Read the model definition and answer for the solid it produces. Units are mm, in the model's axes. Give positions to 0.01 mm unless a question says otherwise; leave off trailing zeros. Order: outer loops, then holes, each group sorted by start corner. A loop starts at its lowest first (then second) coordinate and runs counter-clockwise, first axis right, second up. Notation, with made-up numbers: M 69.25,5 L 99.25,5 A21 cw 99.25,17 Z; hole C 66,36.25 d4. An arc over 180 degrees is marked long. One line per item, written item: value. Start each with the question number.
from build123d import *

# Parameters (mm, degrees)
F0_W     = 33.02
F0_H     = 11.43
F0_R     = 4
F1_DEPTH = 5.08
F2_R     = 2.286
F3_DEPTH = 20.32


with BuildPart() as f1:
    # F0 (on Top) → F1 (new body)
    with BuildSketch(Plane.XY):
        Rectangle(F0_W, F0_H)
        with Locations((-10.2616, 0)):
            Circle(F0_R, mode=Mode.SUBTRACT)
        with Locations((10.2616, 0)):
            Circle(F0_R, mode=Mode.SUBTRACT)
    extrude(amount=F1_DEPTH)

    # F2 (on face) → F3 (join)
    with BuildSketch(Plane(origin=(0, 0, 0), x_dir=(1, 0, 0), z_dir=(0, 0, -1))):
        Circle(F2_R)
    extrude(amount=F3_DEPTH)


solid = f1.part
Q1. Find section B-B, the plane x = 0. Give the vertices of the cut face in (y, z) (3 decimals), then the cut area to 3 significant figures.
Q2. Each of these flat-tipped pins is pushed along its axis until it touches: pin 1 (8 mm diameter, centred on x = -5, z = -13, fed in from +Y); pin 2 (2 mm diameter, centred on y = -0.5, z = -17.5, fed in from -X); pin 3 (6 mm diameter, centred on y = 0.5, z = -5.5, fed in from +X). Where does it stop, or does it pass through?
Q3. Find section D-D, the plane x = -8. Give the vertices of the cut face in (y, z) (3 decimals).
Q4. Determine the mould class of faces 1 (the flat face through (0, 3, 0)), 2 (the cylindrical face through (-0.5, 2.23, -10.02)), 3 (the cylindrical face through (13.957, -1.532, 2.504)) for opening direction X: released by +X, released by -X, zero draft, split by the parting line, or undercut.
Q5. Consider probe 1 along X at (y, z) = (-3, 4.25); probe 2 along Z at (x, y) = (12, -4); probe 3 along Y at (x, z) = (-2, -0.5). Determine where each line is inside the solid, lowest interval first.
Q6. Find section C-C, the plane z = 1.5. Give the vertices of the cut face in (x, y) (3 decimals).
Q7. Find section A-A, the plane y = 0. Give the vertices of the cut face in (x, z), then the cut area to 3 significant figures.
Evaluation:
1. outline: M -5.715,0 L -2.286,0 L -2.286,-20.32 L 2.286,-20.32 L 2.286,0 L 5.715,0 L 5.715,5.08 L -5.715,5.08 Z
1. area: 151 mm2
2. pin 1: y = 2.06
2. pin 2: x = -2.29
2. pin 3: x = 2.29
3. outline: M -5.715,0 L -3.299,0 L -3.299,5.08 L -5.715,5.08 Z; M 3.299,0 L 5.715,0 L 5.715,5.08 L 3.299,5.08 Z
4. face 1: zero draft
4. face 2: split by the parting line
4. face 3: undercut
5. probe 1: -16.51 to -12.91, -7.62 to 7.62, 12.91 to 16.51
5. probe 2: 0 to 5.08
5. probe 3: -1.11 to 1.11
6. outline: M -16.51,-5.715 L 16.51,-5.715 L 16.51,5.715 L -16.51,5.715 Z; hole C -10.262,0 d8; hole C 10.262,0 d8
7. outline: M -16.51,0 L -14.26,0 L -14.26,5.08 L -16.51,5.08 Z; M -6.26,0 L -2.29,0 L -2.29,-20.32 L 2.29,-20.32 L 2.29,0 L 6.26,0 L 6.26,5.08 L -6.26,5.08 Z; M 14.26,0 L 16.51,0 L 16.51,5.08 L 14.26,5.08 Z
7. area: 179 mm2
